```python
from build123d import *

# Parameters (mm, degrees)
PAD_DEPTH    = 0.6
PAD008_DEPTH = 0.6
FILLET_R     = 0.5
SKETCH018_R  = 2.5
PAD009_DEPTH = 1.7
FILLET001_R  = 0.5
SKETCH019_W  = 4
SKETCH019_H  = 2
PAD010_DEPTH = 4


with BuildPart() as part:
    # Sketch → Pad (new body)
    with BuildSketch(Plane.XY):
        with BuildLine():
            ThreePointArc((3.05, 7.6116686738), (-8.2, 0), (3.05, -7.6116686738))
            Line((3.05, 7.6116686738), (3.05, -7.6116686738))
        make_face()
    extrude(amount=-PAD_DEPTH)

    # Sketch017 (on Face4 of Pad) → Pad008 (join)
    with BuildSketch(Plane(origin=(0, 0, -0.6), x_dir=(1, 0, 0), z_dir=(0, 0, -1))):
        with BuildLine():
            ThreePointArc((3.0499999999, 3.3087006514), (-4.5, 0), (3.0499999999, -3.3087006514))
            Line((3.0499999999, 3.3087006514), (3.0499999999, -3.3087006514))
        make_face()
    extrude(amount=PAD008_DEPTH)

    # Fillet
    fillet_edges = [part.edges().sort_by_distance(p)[0] for p in [
        (-4.5, 0, -1.2),
    ]]
    fillet(fillet_edges, radius=FILLET_R)

    # Sketch018 (on Face5 of Fillet) → Pad009 (join)
    with BuildSketch(Plane(origin=(0, 0, -1.2), x_dir=(1, 0, 0), z_dir=(0, 0, -1))):
        Circle(SKETCH018_R)
    extrude(amount=PAD009_DEPTH)

    # Fillet001
    fillet001_edges = [part.edges().sort_by_distance(p)[0] for p in [
        (-2.5, 0, -2.9),
        (-2.5, 0, -1.2),
    ]]
    fillet(fillet001_edges, radius=FILLET001_R)

    # Sketch019 (on Face7 of Fillet001) → Pad010 (join)
    with BuildSketch(Plane(origin=(0, 0, -0.6), x_dir=(1, 0, 0), z_dir=(0, 0, -1))):
        with Locations((0, 6)):
            Rectangle(SKETCH019_W, SKETCH019_H)
        with Locations((0, -6)):
            Rectangle(SKETCH019_W, SKETCH019_H)
    extrude(amount=PAD010_DEPTH)


solid = part.part
```
Read the model definition and answer for the solid it produces. Units are mm, in the model's axes. A direction names the side the tool comes from. Round coordinates to 2 decimals unless told otherwise and drop trailing zeros. Loops run counter-clockwise (first coordinate to the right, second up) from the corner with the lowest first, then second, coordinate; pieces in that order, holes last. Notation, with made-up numbers: (82.5, 12) -> (86.5, 12) arc R31 ccw to (86.5, 46) -> close; hole circle Ø3 at (-7, 72). An arc over 180 degrees is marked (long way). One line per item, written item: value.
1) A cutting plane is placed at C-C (x = -5.25). Determine the outline of the cut face in (y, z).
Answer list:
outline: (-6.3, -0.6) -> (6.3, -0.6) -> (6.3, 0) -> (-6.3, 0) -> close
2) For faces 5 (the face through (2, -6, -3)), 6 (the face through (0, 5, -3)), 7 (the face through (-2, 6, -3)), 8 (the face through (2, 6, -3)), determine the directions among +Z, -Z, +X, -X, +Y, -Y from which every point of the face is accessible in a straight line to the end or side of a thin tool.
Answer list:
face 5: -Z, +X, -Y
face 6: -Z, +X, -X
face 7: -Z, -X, +Y
face 8: -Z, +X, +Y
3) A cutting plane is placed at A-A (z = -4.2). Determine the outline of the cut face in (x, y), and give its area (3 significant figures).
Answer list:
outline: (-2, -7) -> (2, -7) -> (2, -5) -> (-2, -5) -> close; (-2, 5) -> (2, 5) -> (2, 7) -> (-2, 7) -> close
area: 16.0 mm²
4) Flat-ended cylindrical pins translate along their axes: P1, Ø2, axis at y = 6, z = -1.5, coming from the +X side; P2, Ø1.2, axis at x = 1, y = 1, coming from the -Z side; P3, Ø1.6, axis at y = 5.5, z = -2.5, coming from the -X side; P4, Ø1.6, axis at y = -6.5, z = -3.5, coming from the +X side. Find the tip coordinate at first contact, or state that the pin passes through.
Answer list:
P1: stops at x = 3.05
P2: stops at z = -2.9
P3: stops at x = -2
P4: stops at x = 2
5) A cutting plane is placed at B-B (y = 0). Determine the outline of the cut face in (x, z), and give its area (3 significant figures).
Answer list:
outline: (-8.2, -0.6) -> (-4.5, -0.6) -> (-4.5, -0.7) arc R0.5 ccw to (-4, -1.2) -> (-3, -1.2) arc R0.5 cw to (-2.5, -1.7) -> (-2.5, -2.4) arc R0.5 ccw to (-2, -2.9) -> (2, -2.9) arc R0.5 ccw to (2.5, -2.4) -> (2.5, -1.7) arc R0.5 cw to (3, -1.2) -> (3.05, -1.2) -> (3.05, 0) -> (-8.2, 0) -> close
area: 19.7 mm²
6) The mould has two halves that part along Y. Classify faces 1 (the face through (0, 6, -4.6)), 2 (the face through (0, -7, -3)), 3 (the face through (0, 0, -2.9)), 4 (the face through (-8.197, 0.224, -0.296)): pulls with the +Y half, pulls with the -Y half, needs draft (parallel to the pull), parting line crosses it, or undercut.
Answer list:
face 1: needs draft
face 2: pulls with the -Y half
face 3: undercut
face 4: parting line crosses it
7) A cutting plane is placed at D-D (y = 5.5). Determine the outline of the cut face in (x, z).
Answer list:
outline: (-6.08, -0.6) -> (-2, -0.6) -> (-2, -4.6) -> (2, -4.6) -> (2, -0.6) -> (3.05, -0.6) -> (3.05, 0) -> (-6.08, 0) -> close
8) Consider L1, parallel to Y at x = -1.25, z = -1.55; L2, parallel to Y at x = 1.75, z = -4; L3, parallel to Z at x = -3, y = -0.5. Determine where each line is inside the solid, lowest interval first. Write a range as [from, to].
Answer list:
L1: y = [-7, -5], [-2.19, 2.19], [5, 7]
L2: y = [-7, -5], [5, 7]
L3: z = [-1.2, 0]
